```python
from build123d import *

# Parameters (mm, degrees)
SCHNITT_LINEAR_AUSTRAGEN1_DEPTH = 3
M6_GEWINDEBOHRUNG1_D            = 5
M6_GEWINDEBOHRUNG1_DEPTH        = 20
M6_GEWINDEBOHRUNG1_CSINK_D      = 6
M6_GEWINDEBOHRUNG1_CSINK_ANGLE  = 90
M6_GEWINDEBOHRUNG1_TIP          = 1.502151548


with BuildPart() as part:
    # Skizze1 → Rotation1 (revolve)
    with BuildSketch(Plane.XY, mode=Mode.PRIVATE) as rotation1_sk:
        Polygon((-113, 0), (-113, 8.5), (-64, 8.5), (-64, 9.5), (-60, 9.5), (-60, 6), (0, 6), (0, 0), align=None)
    revolve(rotation1_sk.sketch.rotate(Axis((13.513507739, 0, 0), (-1, 0, 0)), 90), axis=Axis((13.513507739, 0, 0), (-1, 0, 0)))

    # Skizze2 → Schnitt-Linear austragen1 (cut)
    with BuildSketch(Plane(origin=(0, 8.5, 0), x_dir=(-1, 0, 0), z_dir=(0, 1, 0))):
        with BuildLine():
            Line((108, 2.5), (97, 2.5))
            ThreePointArc((97, 2.5), (94.5, 0), (97, -2.5))
            Line((97, -2.5), (108, -2.5))
            ThreePointArc((108, -2.5), (110.5, 0), (108, 2.5))
        make_face()
    extrude(amount=-SCHNITT_LINEAR_AUSTRAGEN1_DEPTH, mode=Mode.SUBTRACT)

    # M6 Gewindebohrung1
    with Locations(Plane.ZY.offset(113)):
        with Locations((0, 0)):
            CounterSinkHole(M6_GEWINDEBOHRUNG1_D / 2, M6_GEWINDEBOHRUNG1_CSINK_D / 2, depth=M6_GEWINDEBOHRUNG1_DEPTH, counter_sink_angle=M6_GEWINDEBOHRUNG1_CSINK_ANGLE)
            with Locations((0, 0, -(M6_GEWINDEBOHRUNG1_DEPTH + M6_GEWINDEBOHRUNG1_TIP / 2))):  # 118° drill point
                Cone(0, M6_GEWINDEBOHRUNG1_D / 2, M6_GEWINDEBOHRUNG1_TIP, mode=Mode.SUBTRACT)

    # Skizze31 → Schnitt-Rotation1 (revolve, cut)
    with BuildSketch(Plane(origin=(-60, 0, 0), x_dir=(-1, 0, 0), z_dir=(0, 0, -1)), mode=Mode.PRIVATE) as schnitt_rotation1_sk:
        with BuildLine():
            Line((-4.65055535, 6), (-4.188675135, 5.2))
            ThreePointArc((-4.188675135, 5.2), (-3.822649731, 4.833974596), (-3.322649731, 4.7))
            Line((-3.322649731, 4.7), (-1, 4.7))
            ThreePointArc((-1, 4.7), (-0.292893219, 4.992893219), (0, 5.7))
            Line((0, 5.7), (0, 6))
            Line((0, 6), (-4.65055535, 6))
        make_face()
    revolve(schnitt_rotation1_sk.sketch.rotate(Axis((-73.677186203, 0, 0), (1, 0, 0)), 90), axis=Axis((-73.677186203, 0, 0), (1, 0, 0)), mode=Mode.SUBTRACT)

    # Skizze32 → Schnitt-Rotation11 (revolve, cut)
    with BuildSketch(Plane(origin=(0, 0, 0), x_dir=(0, 0, -1), z_dir=(0, -1, 0)), mode=Mode.PRIVATE) as schnitt_rotation11_sk:
        Polygon((0, -5.351075774), (1.25, -4.6), (1.25, -2.424871131), (2.65, 0), (0, 0), align=None)
    revolve(schnitt_rotation11_sk.sketch.rotate(Axis((0, 0, 0), (-1, 0, 0)), 270), axis=Axis((0, 0, 0), (-1, 0, 0)), mode=Mode.SUBTRACT)


solid = part.part
```
CAD build for the part. Positions are in the model's coordinates, mm. A direction names the side the tool comes from. Round coordinates to 2 decimals unless told otherwise and drop trailing zeros. Write each loop counter-clockwise with the first axis right and the second up, starting at its lowest first coordinate (ties: lowest second). Pieces come first, ordered by that corner, then holes. Notation, with made-up numbers: (7.25, 41) - (52.25, 41) arc R16 ccw to (52.25, 50) - close; hole circle Ø8 at (38.25, 73). An arc over 180 degrees is marked (long way). Return JSON: item names as keys, results as strings. Group by question number.
Item 1: 3-axis set-ups, long thin cutter, end or side, ignore diameter. For faces 4 (the face through (-57.85, 4.59, -1.02)), 5 (the face through (-110.5, 7, -0.1)), 6 (the face through (-102.61, -2.44, 0.54)), 7 (the face through (-3.5, -0.27, 1.22)): which of +Z, -Z, +X, -X, +Y, -Y reach the whole face in a straight line?
Item 2: Band-saw the part on B-B on x = -31.5. List the corners of the cut face in (y, z), plus the area to 3 significant figures.
Item 3: Band-saw the part on A-A on x = -99.5. List the corners of the cut face in (y, z).
Item 4: Probe probe 1 along Y at (x, z) = (-98.5, 0); probe 2 along X at (y, z) = (6, -6.5); probe 3 along X at (y, z) = (-6, 4.75). List the from-to ranges inside material, lowest first.
Item 5: Flat gauge pins, fed straight in: pin 1 Ø4 at (x, z) = (-85.5, -3.5) entering from +Y; pin 2 Ø3 at (x, y) = (-21, 1.5) entering from -Z; pin 3 Ø2 at (y, z) = (-0.5, -0.5) entering from -X. Where does each tip first touch, or does it go through?
Item 6: Mould opens along Z. For faces 1 (the face through (-60, 6, 0)), 2 (the face through (-5.22, -0.05, 0.21)), 3 (the face through (-27.287, -1.802, -5.723)) say: +Z half, -Z half, draft (parallel to the pull), parting line (faces both ways), or undercut.
Resolved:
{
 "1": {"face 4": "none", "face 5": "+Y", "face 6": "-X", "face 7": "+X"},
 "2": {"outline": "circle Ø12 at (0, 0)", "area": "113 mm²"},
 "3": {"outline": "(5.5, -2.5) - (5.5, 2.5) - (8.12, 2.5) arc R8.5 ccw (long way) to (8.12, -2.5) - close; hole circle Ø5 at (0, 0)"},
 "4": {"probe 1": "y = -8.5 to -2.5, 2.5 to 5.5", "probe 2": "x = -64 to -60", "probe 3": "x = -113 to -60"},
 "5": {"pin 1": "stops at y = 8.37", "pin 2": "stops at z = -6", "pin 3": "stops at x = -92.52"},
 "6": {"face 1": "draft", "face 2": "undercut", "face 3": "parting line"}
}
